Geometry: final body of the model. Coordinates: model frame, mm. Give positions to 0.01 mm unless a question says otherwise; leave off trailing zeros. Loops run counter-clockwise (first coordinate to the right, second up) from the corner with the lowest first, then second, coordinate; pieces in that order, holes last. Notation, with made-up numbers: (77, 89.5) - (105, 89.5) arc R36 cw to (105, 126.5) - close; hole circle Ø1 at (-6, 53.25). An arc over 180 degrees is marked (long way). Use CSV: the item, a comma, the result in double quotes. Start each with the question number.
Autodesk Inventor part; units mm, degrees
ref_plane "Start plane" through (0, 0, 0) normal (0, 0, 1) x (1, 0, 0)
ref_plane "End plane" through (0, 0, 1415) normal (0, 0, 1) x (1, 0, 0)
ref_plane "Work Plane4" through (0, -4000, 1415) normal (0, 0, 1) x (1, 0, 0)
ref_plane "Start plane" through (0, 0, 0) normal (0, 0, 1) x (1, 0, 0)
ref_plane "End plane" through (0, 0, 1415) normal (0, 0, 1) x (1, 0, 0)
sketch "Sketch2" plane through (0, 0, 0) normal (0, 0, 1) x (1, 0, 0)
  line L0 (-55, 100.8) -> (-14.95, 100.8)
  line L1 (-55, 110) -> (-55, 100.8)
  line L2 (55, 110) -> (-55, 110)
  line L3 (55, 100.8) -> (55, 110)
  line L4 (14.95, 100.8) -> (55, 100.8)
  line L5 (2.95, -88.8) -> (2.95, 88.8)
  line L6 (55, -100.8) -> (14.95, -100.8)
  line L7 (55, -110) -> (55, -100.8)
  line L8 (-55, -100.8) -> (-55, -110)
  line L9 (-14.95, -100.8) -> (-55, -100.8)
  line L10 (-2.95, 88.8) -> (-2.95, -88.8)
  line L11 (0, -154) -> (0, 154) construction
  line L12 (-2.95, -100.8) -> (2.95, -100.8) construction
  arc A0 (-14.95, -100.8) -> (-2.95, -88.8) centre (-14.95, -88.8) ccw
  arc A1 (-2.95, 88.8) -> (-14.95, 100.8) centre (-14.95, 88.8) ccw
  arc A2 (14.95, 100.8) -> (2.95, 88.8) centre (14.95, 88.8) ccw
  arc A3 (2.95, -88.8) -> (14.95, -100.8) centre (14.95, -88.8) ccw
  line L13 (-77, 0) -> (77, 0) construction
  line L14 (-55, -110) -> (55, -110)
  point P0 (-2.95, 100.8)
  point P1 (2.95, 100.8)
  point P2 (0, 0)
  point P3 (0, -100.8)
  point P4 (0, 0)
  dimension "d1" = 220
  dimension "d3" = 9.2
  dimension "d5" = 5.9
  dimension "d7" = 110
  dimension "d13" = 12
  dimension "d14" = 110
  dimension "d15" = 55
extrude "Body" add sketch "Sketch2" along normal up to surface (1415 mm away) from surface at 0
sketch "Sketch3" plane through (0, 0, 0) normal (0, 0, 1) x (1, 0, 0)
  line L0 (0, 0) -> (10, 0)
ref_plane "Work Plane3" through (0, 0, 0) normal (0, -1, 0) x (1, 0, 0)
ref_plane "Work Plane4" through (0, -4000, 1415) normal (0, 0, 1) x (1, 0, 0)
split "Split1" plane through (0, -4000, 1415) removes the side toward (0, 0, 1)
sketch "Sketch4" plane through (0, 0, 0) normal (0, -1, 0) x (1, 0, 0)
  line L0 (-2, 0) -> (12, 0)
  line L1 (-2, 1415) -> (12, 1415)
  dimension "d19" = 1415
equation "\"d1\" = ParH"
equation "\"d3\" = t2"
equation "\"d7\" = b"
equation "\"d13\" = R1"
equation "\"d14\" = 0.5 * d1"
equation "\"d15\" = 0.5 * d7"
equation "\"d8\" = G_L"
equation "\"b\" = 110"
equation "\"ParH\" = 220"
equation "\"R1\" = 12"
equation "\"G_L\" = d19"
equation "\"t1\" = 5.9"
equation "\"t2\" = 9.2"
equation "\"G_OFFSET_START\" = 0"
equation "\"G_OFFSET_END\" = -85"
equation "\"d17\" = G_OFFSET_END + B_L"
properties part number "DIN 1025 - IPE 220-1415" material "Steel, Mild"
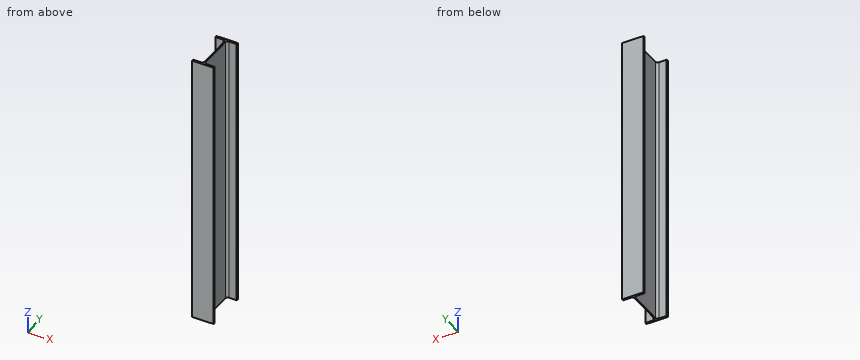
Item 1: Section B-B (z = 890). Output: boundary loops of the cut face in (x, y), plus the area to 3 significant figures.
Item 2: Ray query, probe 1 along Y at (x, z) = (-43, 925.5); probe 2 along X at (y, z) = (1.5, 1314.5); probe 3 along Y at (x, z) = (11, 1120). Return the intervals inside material, ascending.
Item 3: Section C-C (y = 69). Output: boundary loops of the cut face in (x, z), plus the area to 3 significant figures.
Item 4: Section A-A (x = 32.5). Output: boundary loops of the cut face in (y, z), plus the area to 3 significant figures.
Item 5: Pin query (flat end, axial travel): pin 1 Ø12 at (y, z) = (-77.5, 151.5) entering from +X. Return the tip coordinate at first contact, or that it passes through.
Outcome:
1,outline,"(-55, -110) - (55, -110) - (55, -100.8) - (14.95, -100.8) arc R12 cw to (2.95, -88.8) - (2.95, 88.8) arc R12 cw to (14.95, 100.8) - (55, 100.8) - (55, 110) - (-55, 110) - (-55, 100.8) - (-14.95, 100.8) arc R12 cw to (-2.95, 88.8) - (-2.95, -88.8) arc R12 cw to (-14.95, -100.8) - (-55, -100.8) - close"
1,area,"3,340 mm2"
2,probe 1,"y = -110 to -100.8, 100.8 to 110"
2,probe 2,"x = -2.95 to 2.95"
2,probe 3,"y = -110 to -100.13, 100.13 to 110"
3,outline,"(-2.95, 0) - (2.95, 0) - (2.95, 1415) - (-2.95, 1415) - close"
3,area,"8,350 mm2"
4,outline,"(-110, 0) - (-100.8, 0) - (-100.8, 1415) - (-110, 1415) - close; (100.8, 0) - (110, 0) - (110, 1415) - (100.8, 1415) - close"
4,area,"26,000 mm2"
5,pin 1,"stops at x = 2.95"
